from build123d import *

# Parameters (mm, degrees)
F3_DEPTH = 1.5
F4_R     = 3.25
F5_DEPTH = 3
F6_COUNT = 2
F7_R     = 3.25
F8_DEPTH = 25


with BuildPart() as f3:
    # F2 (on Front) → F3 (new body, symmetric)
    with BuildSketch(Plane.XZ):
        with BuildLine():
            Line((-5.9866518188, 30.4), (-7.9822024251, 0.5333333333))
            ThreePointArc((-7.9822024251, 0.5333333333), (0, -8), (7.9822024251, 0.5333333333))
            Line((7.9822024251, 0.5333333333), (5.9866518188, 30.4))
            ThreePointArc((5.9866518188, 30.4), (0, 36), (-5.9866518188, 30.4))
        make_face()
    extrude(amount=F3_DEPTH, both=True)

    # F4 (on face) → F5 (cut, through all)
    with BuildSketch(Plane.XZ.offset(1.5)):
        with Locations((0, 30)):
            Circle(F4_R)
    extrude(amount=-F5_DEPTH, mode=Mode.SUBTRACT)

    # F6: F3 ×2 about axis
    f6_axis = Axis((0, 0, 0), (0, -1, 0))


with BuildPart() as f3_1:
    add(f3.part)
    for i in range(1, F6_COUNT):
        add(f3.part.rotate(f6_axis, i * 360 / F6_COUNT))

    # F7 (on face) → F8 (cut)
    with BuildSketch(Plane.XZ.offset(1.5)):
        Circle(F7_R)
    extrude(amount=-F8_DEPTH, mode=Mode.SUBTRACT)


solid = f3_1.part
Part model, mm, in its own coordinate system. Give positions to 0.01 mm unless a question says otherwise; leave off trailing zeros. Write each loop counter-clockwise with the first axis right and the second up, starting at its lowest first coordinate (ties: lowest second). Pieces come first, ordered by that corner, then holes.
1) Cut at D-D on z = -11. Write the cut outline in (x, y), then the cut area to 3 significant figures.
Resolved:
outline: (-7.28, -1.5) - (7.28, -1.5) - (7.28, 1.5) - (-7.28, 1.5) - close
area: 43.7 mm2
2) Cut at A-A on x = 0. Write the cut outline in (y, z), then the cut area to 4 significant figures.
Resolved:
outline: (-1.5, -36) - (1.5, -36) - (1.5, -33.25) - (-1.5, -33.25) - close; (-1.5, -26.75) - (1.5, -26.75) - (1.5, -3.25) - (-1.5, -3.25) - close; (-1.5, 3.25) - (1.5, 3.25) - (1.5, 26.75) - (-1.5, 26.75) - close; (-1.5, 33.25) - (1.5, 33.25) - (1.5, 36) - (-1.5, 36) - close
area: 157.5 mm2
3) Probe L1, parallel to Z at x = 0, y = 0.85; L2, parallel to Z at x = 1.5, y = 0.9; L3, parallel to X at y = -0.5, z = 27. List the from-to ranges inside material, lowest first.
Resolved:
L1: z = -36 to -33.25, -26.75 to -3.25, 3.25 to 26.75, 33.25 to 36
L2: z = -35.81 to -32.88, -27.12 to -2.88, 2.88 to 27.12, 32.88 to 35.81
L3: x = -6.21 to -1.25, 1.25 to 6.21
4) Pin check, flat tips, straight feed: pin 1 (6 mm diameter, centred on x = 0, z = 30, fed in from -Y); pin 2 (1.5 mm diameter, centred on y = -0.5, z = -13.5, fed in from +X); pin 3 (1 mm diameter, centred on y = 1, z = 9, fed in from -X). Stop position of each tip, or through.
Resolved:
pin 1: passes through
pin 2: stops at x = 7.17
pin 3: stops at x = -7.45
5) Cut at B-B on y = 0.45. Write the cut outline in (x, z), then the cut area to 3 significant figures.
Resolved:
outline: (-7.98, -0.53) - (-5.99, -30.4) arc R6 ccw to (5.99, -30.4) - (7.98, -0.53) arc R8 ccw to (7.98, 0.53) - (5.99, 30.4) arc R6 ccw to (-5.99, 30.4) - (-7.98, 0.53) arc R8 ccw to start; hole circle Ø6.5 at (0, -30); hole circle Ø6.5 at (0, 0); hole circle Ø6.5 at (0, 30)
area: 855 mm2
6) Cut at C-C on z = -31. Write the cut outline in (x, y).
Resolved:
outline: (-5.92, -1.5) - (-3.09, -1.5) - (-3.09, 1.5) - (-5.92, 1.5) - close; (3.09, -1.5) - (5.92, -1.5) - (5.92, 1.5) - (3.09, 1.5) - close
7) Two-plate mould, pull along X, no slides. Class faces 1 (the face through (6.97, -0.02, -15.68)), 2 (the face through (-7, -0.02, -15.26)), 3 (the face through (-0.705, -0.021, 26.827)), 4 (the face through (-2.579, -0.021, -1.978)): released by +X, released by -X, zero draft, split by the parting line, or undercut.
Resolved:
face 1: released by +X
face 2: released by -X
face 3: undercut
face 4: undercut
